```python
from build123d import *

# Parameters (mm, degrees)
SKETCH1_W                          = 152
SKETCH1_H                          = 86
BOSS_EXTRUDE1_DEPTH                = 10
SKETCH2_W                          = 152
SKETCH2_H                          = 86
SKETCH2_W_2                        = 142
SKETCH2_H_2                        = 76
BOSS_EXTRUDE2_DEPTH                = 10
F_2_0350_40_UNS_TAPPED_HOLE1_D     = 50.955575
F_2_0350_40_UNS_TAPPED_HOLE1_DEPTH = 106.56


with BuildPart() as part:
    # Sketch1 → Boss-Extrude1 (new body)
    with BuildSketch(Plane(origin=(0, 0, 0), x_dir=(1, 0, 0), z_dir=(0, 1, 0))):
        Rectangle(SKETCH1_W, SKETCH1_H)
    extrude(amount=BOSS_EXTRUDE1_DEPTH)

    # Sketch2 → Boss-Extrude2 (add)
    with BuildSketch(Plane(origin=(0, 10, 0), x_dir=(1, 0, 0), z_dir=(0, 1, 0))):
        Rectangle(SKETCH2_W, SKETCH2_H)
        Rectangle(SKETCH2_W_2, SKETCH2_H_2, mode=Mode.SUBTRACT)
    extrude(amount=BOSS_EXTRUDE2_DEPTH)

    # 2.0350-40 UNS Tapped Hole1
    with Locations(Plane(origin=(0, 0, 0), x_dir=(-1, 0, 0), z_dir=(0, -1, 0))):
        with Locations((0, 0)):
            Hole(F_2_0350_40_UNS_TAPPED_HOLE1_D / 2, depth=F_2_0350_40_UNS_TAPPED_HOLE1_DEPTH)


solid = part.part
```
For this review, take the finished solid that the model builds, in its own axes (mm). A direction names the side the tool comes from. Coordinates: 2 decimals unless noted, no trailing zeros. Order: outer loops, then holes, each group sorted by start corner. A loop starts at its lowest first (then second) coordinate and runs counter-clockwise, first axis right, second up. Notation, with made-up numbers: (48, 77) -> (63, 77) arc R18 cw to (63, 102) -> close; hole circle Ø7 at (28, -10). An arc over 180 degrees is marked (long way). Use CSV: the item, a comma, the result in double quotes. Start each with the question number.
Item 1: We need section A-A, the plane x = 0. Give the boundary of the cut face in (y, z), then the cut area to 3 significant figures.
Item 2: For faces 1 (the face through (-1, 10, -26)), 2 (the face through (0, 20, 41)), list the 3-axis set-ups (+Z, -Z, +X, -X, +Y, -Y) from which the entire face can be reached by the end or side of a thin tool; tool diameter is ignored.
Item 3: We need section B-B, the plane z = 0. Give the boundary of the cut face in (x, y), then the cut area to 3 significant figures.
Item 4: We need section D-D, the plane x = 61.5. Give the boundary of the cut face in (y, z).
Item 5: Draft analysis for pull direction X (two halves, no side actions). For faces 3 (the face through (-71, 15, 1)), 4 (the face through (-76, 10, 1)), 5 (the face through (-1, 10, 43)), state which applies: pulls with the +X half, pulls with the -X half, needs draft (parallel to the pull), parting line crosses it, or undercut.
Item 6: Wall thickness on probe 1 along Z at (x, y) = (0, 4.25); probe 2 along Z at (x, y) = (38, 13.5); probe 3 along X at (y, z) = (18.75, 2.5): over which ranges is each line inside the solid? List them lowest first.
Item 7: We need section C-C, the plane y = 6.5. Give the boundary of the cut face in (x, z), then the cut area to 3 significant figures.
Item 8: Insertion check: pin 1 (23 mm diameter, centred on x = -14, z = -3.5, fed in from +Y). The pin has a flat end and moves straight along its axis. Give the tip position at first contact, or say it passes through.
Derived:
1,outline,"(0, -43) -> (20, -43) -> (20, -38) -> (10, -38) -> (10, -25.48) -> (0, -25.48) -> close; (0, 25.48) -> (10, 25.48) -> (10, 38) -> (20, 38) -> (20, 43) -> (0, 43) -> close"
1,area,"450 mm^2"
2,face 1,"+Y"
2,face 2,"+Z, -Z, +X, -X, +Y"
3,outline,"(-76, 0) -> (-25.48, 0) -> (-25.48, 10) -> (-71, 10) -> (-71, 20) -> (-76, 20) -> close; (25.48, 0) -> (76, 0) -> (76, 20) -> (71, 20) -> (71, 10) -> (25.48, 10) -> close"
3,area,"1,110 mm^2"
4,outline,"(0, -43) -> (20, -43) -> (20, -38) -> (10, -38) -> (10, 38) -> (20, 38) -> (20, 43) -> (0, 43) -> close"
5,face 3,"undercut"
5,face 4,"pulls with the -X half"
5,face 5,"needs draft"
6,probe 1,"z = -43 to -25.48, 25.48 to 43"
6,probe 2,"z = -43 to -38, 38 to 43"
6,probe 3,"x = -76 to -71, 71 to 76"
7,outline,"(-76, -43) -> (76, -43) -> (76, 43) -> (-76, 43) -> close; hole circle Ø50.96 at (0, 0)"
7,area,"11,000 mm^2"
8,pin 1,"stops at y = 10"
